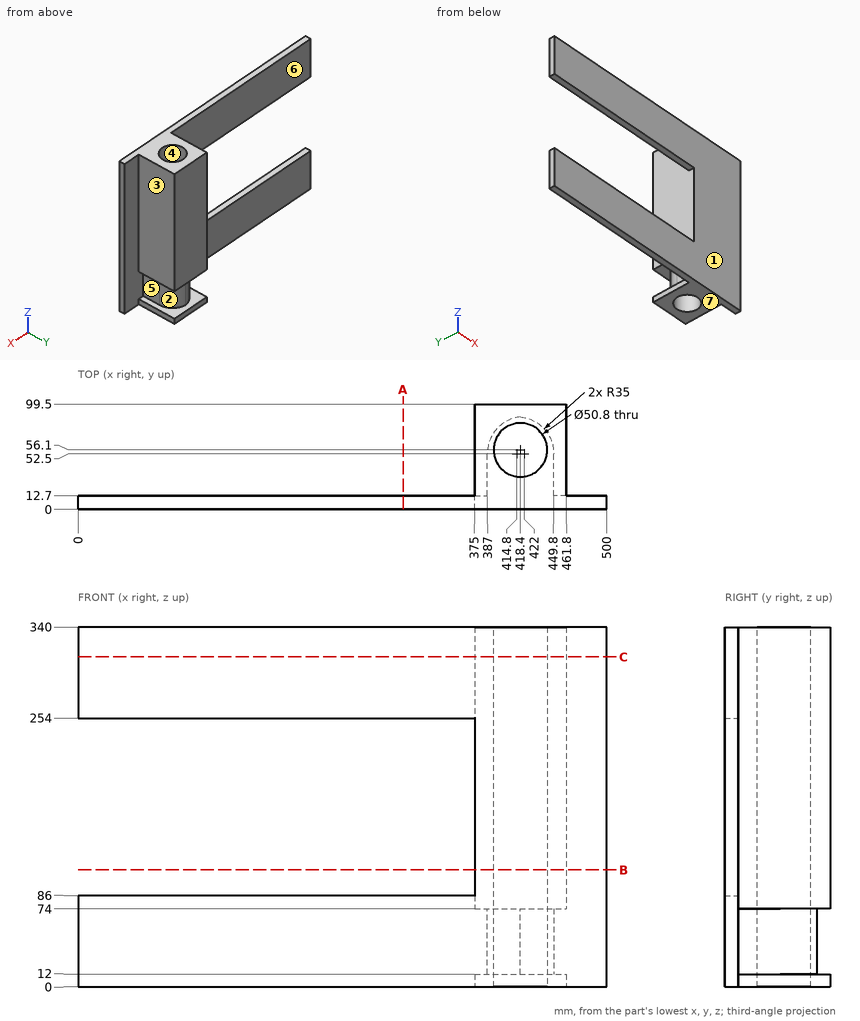
Job drawing, mm, ordinate dimensions from the low corner. One solid piece. A direction names the side the tool comes from. Round coordinates to 2 decimals unless told otherwise and drop trailing zeros. Order: outer loops, then holes, each group sorted by start corner. A loop starts at its lowest first (then second) coordinate and runs counter-clockwise, first axis right, second up. Notation, with made-up numbers: M 74,25 L 115,25 A25 cw 115,53 Z; hole C 70.25,40 d4. An arc over 180 degrees is marked long. Write each question's results on one line, items separated by ' | '. Start each with the question number.
(1) Probe probe 1 along Y at (x, z) = (418.4, 138.5); probe 2 along X at (y, z) = (56, 182); probe 3 along Z at (x, y) = (70.5, 11.5). List the from-to ranges inside material, lowest first. Write a range as from..to.
(2) Saw through at C-C, the plane z = 312. Give the cut face in (x, y).
(3) Drop flat-ended pins along their axis: pin 1 (3 mm diameter, centred on y = 31.5, z = 34, fed in from -X); pin 2 (9.5 mm diameter, centred on y = 76, z = 3.5, fed in from -X); pin 3 (9.5 mm diameter, centred on y = 77, z = 3.5, fed in from +X). Give the stop position or say it passes through.
(4) Which spindle directions (+Z, -Z, +X, -X, +Y, -Y) get a long thin tool onto all of the face, cutting with end or side? Do the marked faces 5, 6 and 7. Say none if no direction does.
(5) Saw through at B-B, the plane z = 110.5. Give the cut face in (x, y).
(6) Saw through at A-A, the plane x = 307.5. Give the cut face in (y, z), then the cut area to 3 significant figures.
(7) Two-plate mould, pull along Y, no slides. Class the marked faces 1, 2, 3 and 4: pulls with the +Y half, pulls with the -Y half, needs draft (parallel to the pull), parting line crosses it, or undercut.
Established:
1) probe 1: y = 0..30.7, 81.5..99.5 | probe 2: x = 375..393, 443.8..461.8 | probe 3: z = 0..86, 254..340
2) outline: M 0,0 L 500,0 L 500,12.7 L 461.8,12.7 L 461.8,99.5 L 375,99.5 L 375,12.7 L 0,12.7 Z; hole C 418.4,56.1 d50.8
3) pin 1: stops at x = 387 | pin 2: stops at x = 375 | pin 3: stops at x = 461.8
4) face 5: +X, +Y | face 6: +Z, -Z, -X, +Y | face 7: -Z, +X, -X, +Y, -Y
5) outline: M 375,0 L 500,0 L 500,12.7 L 461.8,12.7 L 461.8,99.5 L 375,99.5 Z; hole C 418.4,56.1 d50.8
6) outline: M 0,0 L 12.7,0 L 12.7,86 L 0,86 Z; M 0,254 L 12.7,254 L 12.7,340 L 0,340 Z | area: 2,180 mm^2
7) face 1: pulls with the -Y half | face 2: pulls with the +Y half | face 3: needs draft | face 4: undercut
